Could you check a few things on this model? Use its own coordinates, in mm. A direction names the side the tool comes from. Round coordinates to 2 decimals unless told otherwise and drop trailing zeros. Write each loop counter-clockwise with the first axis right and the second up, starting at its lowest first coordinate (ties: lowest second). Pieces come first, ordered by that corner, then holes.
```python
from build123d import *

# Parameters (mm, degrees)
F0_W     = 25.4
F0_H     = 25.4
F1_DEPTH = 25.4
F2_W     = 2.275166
F2_H     = 10.333045
F2_R     = 3.687408
F3_DEPTH = 15.494
F4_R     = 5.08
F5_R     = 1.27
F6_R     = 0.254


with BuildPart() as f1:
    # F0 (on Front) → F1 (new body)
    with BuildSketch(Plane.XZ):
        Rectangle(F0_W, F0_H)
    extrude(amount=F1_DEPTH)

    # F2 (on face) → F3 (cut)
    with BuildSketch(Plane.XZ.offset(25.4)):
        with Locations((-7.583885, 5.166523)):
            Rectangle(F2_W, F2_H)
        with Locations((7.583885, 5.166523)):
            Rectangle(F2_W, F2_H)
        with Locations((0, -5.782713)):
            Circle(F2_R)
    extrude(amount=-F3_DEPTH, mode=Mode.SUBTRACT)

    # F4
    f4_edges = [f1.edges().sort_by_distance(p)[0] for p in [
        (-12.7, -12.7, 12.7),
        (12.7, -12.7, 12.7),
        (-12.7, -12.7, -12.7),
        (12.7, -12.7, -12.7),
    ]]
    fillet(f4_edges, radius=F4_R)

    # F5
    f5_edges = [f1.edges().sort_by_distance(p)[0] for p in [
        (0, 0, 12.7),
        (11.212102, 0, 11.212102),
        (-11.212102, 0, 11.212102),
        (12.7, 0, 0),
        (-12.7, 0, 0),
        (11.212102, 0, -11.212102),
        (-11.212102, 0, -11.212102),
        (0, 0, -12.7),
    ]]
    fillet(f5_edges, radius=F5_R)

    # F6
    f6_edges = [f1.edges().sort_by_distance(p)[0] for p in [
        (0, -25.4, 12.7),
        (11.212102, -25.4, 11.212102),
        (-11.212102, -25.4, 11.212102),
        (12.7, -25.4, 0),
        (-12.7, -25.4, 0),
        (11.212102, -25.4, -11.212102),
        (-11.212102, -25.4, -11.212102),
        (0, -25.4, -12.7),
        (-3.687408, -25.4, -5.782713),
        (-8.721468, -25.4, 5.166523),
        (-7.583885, -25.4, 0),
        (-6.446302, -25.4, 5.166523),
        (-7.583885, -25.4, 10.333045),
        (7.583885, -25.4, 10.333045),
        (6.446302, -25.4, 5.166523),
        (7.583885, -25.4, 0),
        (8.721468, -25.4, 5.166523),
    ]]
    fillet(f6_edges, radius=F6_R)


solid = f1.part
```
Q1. Imagine slicing it at C-C, the plane y = -11. Write out the boundary of the cut face in (x, z).
Q2. We'd pull the mould along Z, two halves only. Please class faces 3 (the flat face through (12.7, -13, 0)), 4 (the flat face through (0, -13, 12.7)), 5 (the flat face through (8, -18, 0)): pulls with the +Z half, pulls with the -Z half, needs draft (parallel to the pull), parting line crosses it, or undercut.
Q3. If I drill on L1, parallel to X at y = -13.75, z = 7.5; L2, parallel to Z at x = -6.5, y = -20.5; L3, parallel to Z at x = 0, y = -14.25, over which ranges is the centre line in solid material (lowest first)?
Q4. On a 3-axis mill with a long thin cutter (end or side, diameter ignored), from which of +Z, -Z, +X, -X, +Y, -Y can I reach the whole of each face in a straight line? I mean faces 1 (the flat face through (6.446, -18, 5)), 2 (the cylindrical face through (-0.107, -0.362, -12.318)). Say none if no direction works.
Q5. Imagine slicing it at B-B, the plane x = 0. Write out the boundary of the cut face in (y, z), then the cut area to 3 significant figures.
Q6. I'm going to push a flat-ended pin straight in: pin 1 Ø1.1 at (x, z) = (8, 5.5) entering from -Y. Where does the tip first touch, or does it pass through?
Q7. Imagine slicing it at A-A, the plane y = -4.5. Write out the boundary of the cut face in (x, z), then the cut area to 3 significant figures.
Results found:
1. outline: (-12.7, -7.62) arc R5.08 ccw to (-7.62, -12.7) - (7.62, -12.7) arc R5.08 ccw to (12.7, -7.62) - (12.7, 7.62) arc R5.08 ccw to (7.62, 12.7) - (-7.62, 12.7) arc R5.08 ccw to (-12.7, 7.62) - close; hole (-8.72, 0) - (-6.45, 0) - (-6.45, 10.33) - (-8.72, 10.33) - close; hole circle Ø7.37 at (0, -5.78); hole (6.45, 0) - (8.72, 0) - (8.72, 10.33) - (6.45, 10.33) - close
2. face 3: needs draft
2. face 4: pulls with the +Z half
2. face 5: undercut
3. L1: x = -12.7 to -8.72, -6.45 to 6.45, 8.72 to 12.7
3. L2: z = -12.7 to 0, 10.33 to 12.7
3. L3: z = -12.7 to -9.47, -2.1 to 12.7
4. face 1: -Y
4. face 2: -Z, +X, -X, +Y
5. outline: (-25.4, -12.45) arc R0.25 ccw to (-25.15, -12.7) - (-1.27, -12.7) arc R1.27 ccw to (0, -11.43) - (0, 11.43) arc R1.27 ccw to (-1.27, 12.7) - (-25.15, 12.7) arc R0.25 ccw to (-25.4, 12.45) - (-25.4, -1.84) arc R0.25 ccw to (-25.15, -2.1) - (-9.91, -2.1) - (-9.91, -9.47) - (-25.15, -9.47) arc R0.25 ccw to (-25.4, -9.72) - close
5. area: 530 mm2
6. pin 1: stops at y = -9.91
7. outline: (-12.7, -7.62) arc R5.08 ccw to (-7.62, -12.7) - (7.62, -12.7) arc R5.08 ccw to (12.7, -7.62) - (12.7, 7.62) arc R5.08 ccw to (7.62, 12.7) - (-7.62, 12.7) arc R5.08 ccw to (-12.7, 7.62) - close
7. area: 623 mm2
